Design review of the part shown in the three views and the two pictorial views. Dimensions are in mm from the part's minimum x, y and z. A direction names the side the tool comes from. Coordinates: 2 decimals unless noted, no trailing zeros. Write each loop counter-clockwise with the first axis right and the second up, starting at its lowest first coordinate (ties: lowest second). Pieces come first, ordered by that corner, then holes.
Q1. For the marked faces 1, 2, 3 and 4, list the 3-axis set-ups (+Z, -Z, +X, -X, +Y, -Y) from which the entire face can be reached by the end or side of a thin tool; tool diameter is ignored.
Q2. Take a section at A-A, the plane z = 1. Write out the cut boundary in (x, y).
Q3. Take a section at B-B, the plane y = 3.25. Write out the cut boundary in (x, z).
Q4. For pin 1 Ø2 at (x, z) = (36.5, 2.5) entering from +Y; pin 2 Ø1.9 at (x, z) = (3, 4.5) entering from +Y; pin 3 Ø1.9 at (x, z) = (41.5, 3) entering from -Y, all flat-tipped, find the tip position at first contact; note any pin that passes through.
Q5. Take a section at C-C, the plane x = 34. Write out the cut boundary in (y, z), plus the area to 3 significant figures.
Q6. For L1, parallel to Y at x = 4, z = 4.5; L2, parallel to X at y = 17.25, z = 3.25; L3, parallel to X at y = 16.25, z = 4, list the stretches that pass through material, from the lowest coordinate up.
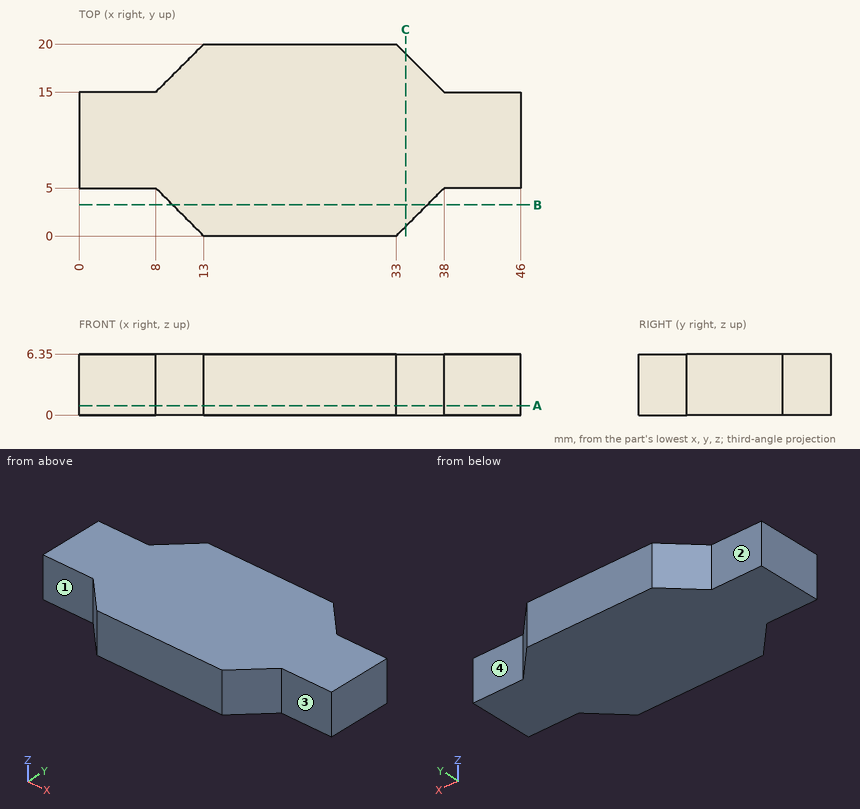
Responses:
1. face 1: +Z, -Z, -X, -Y
1. face 2: +Z, -Z, -X, +Y
1. face 3: +Z, -Z, +X, -Y
1. face 4: +Z, -Z, +X, +Y
2. outline: (0, 5) - (8, 5) - (13, 0) - (33, 0) - (38, 5) - (46, 5) - (46, 15) - (38, 15) - (33, 20) - (13, 20) - (8, 15) - (0, 15) - close
3. outline: (9.75, 0) - (36.25, 0) - (36.25, 6.35) - (9.75, 6.35) - close
4. pin 1: stops at y = 17.5
4. pin 2: stops at y = 15
4. pin 3: stops at y = 5
5. outline: (1, 0) - (19, 0) - (19, 6.35) - (1, 6.35) - close
5. area: 114 mm2
6. L1: y = 5 to 15
6. L2: x = 10.25 to 35.75
6. L3: x = 9.25 to 36.75
